```python
from build123d import *

# Parameters (mm, degrees)
PAD_DEPTH       = 980
POCKET_DEPTH    = 59.501
POCKET001_DEPTH = 59.501


with BuildPart() as part:
    # Sketch → Pad (new body)
    with BuildSketch(Plane.XY):
        Polygon((-29.75, 25), (-29.75, 0), (29.75, 0), (29.75, 25), (28.583333, 25), (28.583333, 1.166667), (0.583333, 1.166667), (0.583333, 25), (-0.583333, 25), (-0.583333, 1.166667), (-28.583333, 1.166667), (-28.583333, 25), align=None)
    extrude(amount=PAD_DEPTH)

    # Sketch001 (on Face3 of Pad) → Pocket (cut, through all)
    with BuildSketch(Plane.YZ.offset(29.75)):
        Polygon((0, 0), (25, 25), (25, 0), align=None)
    extrude(amount=-POCKET_DEPTH, mode=Mode.SUBTRACT)

    # Sketch002 (on Face6 of Pocket) → Pocket001 (cut, through all)
    with BuildSketch(Plane.YZ.offset(29.75)):
        Polygon((0, 980), (25, 955), (25, 980), align=None)
    extrude(amount=-POCKET001_DEPTH, mode=Mode.SUBTRACT)


solid = part.part
```
Source: CAD feature listing. Evaluate the final solid. Frame: model axes, mm. A direction names the side the tool comes from. Round coordinates to 2 decimals unless told otherwise and drop trailing zeros. Loops run counter-clockwise (first coordinate to the right, second up) from the corner with the lowest first, then second, coordinate; pieces in that order, holes last. Notation, with made-up numbers: M 70,42 L 112,42 A21 cw 112,81 Z; hole C 22,20.25 d8. An arc over 180 degrees is marked long. Use a Markdown table: item, result. Add a question column.
1. Section query B-B on z = 385.5. Return the cut outline in (x, y).
2. Line query: line 1 (X direction, y = 9, z = 660); line 2 (Y direction, x = -26.5, z = 473.5). Output: solid intervals per line, ascending.
3. Section query A-A on y = 9.5. Return the cut outline in (x, z), then the cut area to 3 significant figures.
4. Mould query, pull axis X, two halves, no side actions, for faces 1 (the flat face through (0, 9, 971)), 2 (the flat face through (29.75, 12, 483)), 3 (the flat face through (-14, 1.167, 483)). Classes: pulls with the +X half, pulls with the -X half, needs draft (parallel to the pull), parting line crosses it, or undercut.
5. Reachability of faces 4 (the flat face through (0, 9, 9)), 5 (the flat face through (15, 1.167, 483)) from +Z, -Z, +X, -X, +Y, -Y: full face, straight path, thin tool, end or side. Return the list, or none.
6. Contact query for a flat-ended pin moving along its axis: P1, Ø14, axis at x = 17.5, z = 686.5, coming from the +Y side. Output: stop coordinate, or through.
7. Section query C-C on x = -18. Return the cut outline in (y, z).
Reported:
| question | item | result |
|---|---|---|
| 1 | outline | M -29.75,0 L 29.75,0 L 29.75,25 L 28.58,25 L 28.58,1.17 L 0.58,1.17 L 0.58,25 L -0.58,25 L -0.58,1.17 L -28.58,1.17 L -28.58,25 L -29.75,25 Z |
| 2 | line 1 | x = -29.75 to -28.58, -0.58 to 0.58, 28.58 to 29.75 |
| 2 | line 2 | y = 0 to 1.17 |
| 3 | outline | M -29.75,9.5 L -28.58,9.5 L -28.58,970.5 L -29.75,970.5 Z; M -0.58,9.5 L 0.58,9.5 L 0.58,970.5 L -0.58,970.5 Z; M 28.58,9.5 L 29.75,9.5 L 29.75,970.5 L 28.58,970.5 Z |
| 3 | area | 3,360 mm² |
| 4 | face 1 | needs draft |
| 4 | face 2 | pulls with the +X half |
| 4 | face 3 | undercut |
| 5 | face 4 | -Z, +X, -X, +Y |
| 5 | face 5 | +Z, -Z, +Y |
| 6 | P1 | stops at y = 1.17 |
| 7 | outline | M 0,0 L 1.17,1.17 L 1.17,978.83 L 0,980 Z |
